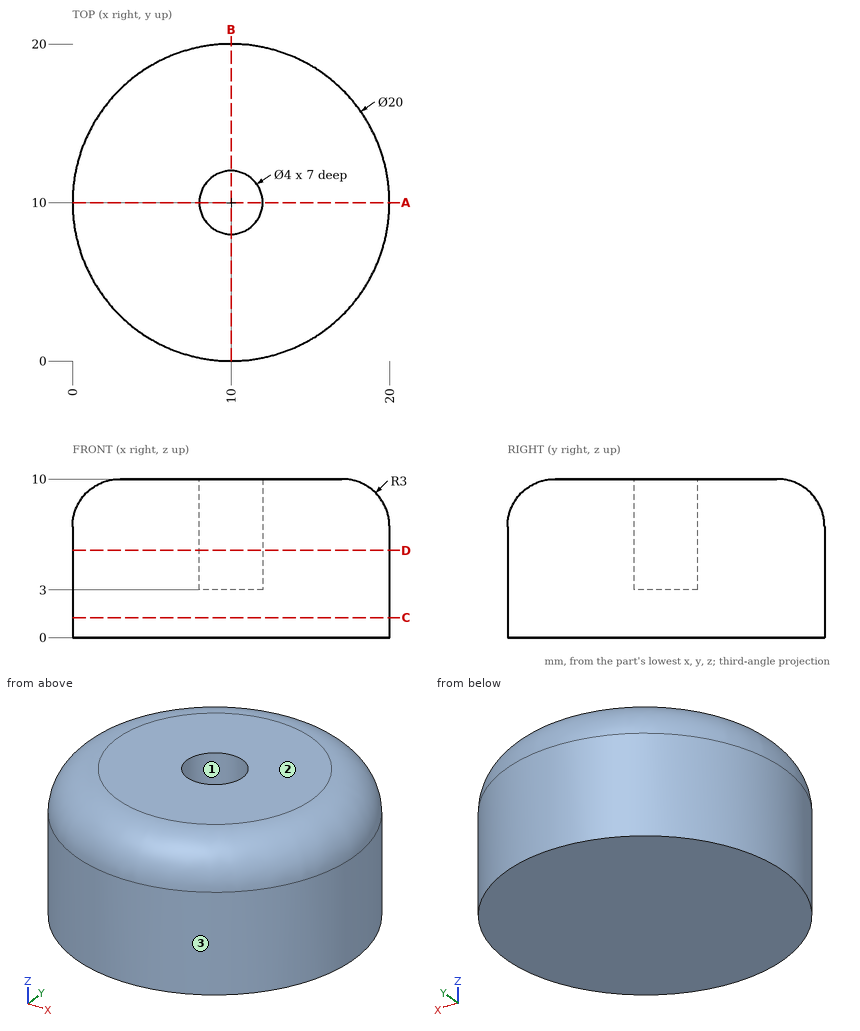
The figure shows three views and two pictorial views of one solid part (mm, origin at its lowest corner). Answer the questions. Round coordinates to 2 decimals unless told otherwise and drop trailing zeros. Write each loop counter-clockwise with the first axis right and the second up, starting at its lowest first coordinate (ties: lowest second). Pieces come first, ordered by that corner, then holes. Notation, with made-up numbers: M 49.5,34 L 60.5,34 A26 cw 60.5,51 Z; hole C -32.75,29.25 d3. An arc over 180 degrees is marked long. Use a Markdown table: item, result.
1) Consider line 1 (Y direction, x = 10, z = 4.5); line 2 (Y direction, x = 10, z = 8.5); line 3 (X direction, y = 9.75, z = 8.25). Determine where each line is inside the solid, lowest interval first. Write a range as [from, to].
Taken from the geometry:
| item | result |
|---|---|
| line 1 | y = [0, 8], [12, 20] |
| line 2 | y = [0.4, 8], [12, 19.6] |
| line 3 | x = [0.28, 8.02], [11.98, 19.72] |
2) The part is cut by section C-C on z = 1.25. Give the vertices of the cut face in (x, y), plus the area to 3 significant figures.
Taken from the geometry:
| item | result |
|---|---|
| outline | C 10,10 d20 |
| area | 314 mm2 |
3) Flat-ended cylindrical pins translate along their axes: pin 1 (10 mm diameter, centred on x = 14.5, y = 4.5, fed in from -Z); pin 2 (1 mm diameter, centred on y = 8, z = 1.5, fed in from -X); pin 3 (5 mm diameter, centred on x = 4, z = 2.5, fed in from +Y); pin 4 (6 mm diameter, centred on x = 5, z = 6.5, fed in from +Y). Find the tip coordinate at first contact, or state that the pin passes through.
Taken from the geometry:
| item | result |
|---|---|
| pin 1 | stops at z = 0 |
| pin 2 | stops at x = 0.11 |
| pin 3 | stops at y = 19.37 |
| pin 4 | stops at y = 19.8 |
4) Determine the mould class of the marked faces 1, 2 and 3 for opening direction X: pulls with the +X half, pulls with the -X half, needs draft (parallel to the pull), parting line crosses it, or undercut.
Taken from the geometry:
| item | result |
|---|---|
| face 1 | undercut |
| face 2 | needs draft |
| face 3 | parting line crosses it |
5) The part is cut by section A-A on y = 10. Give the vertices of the cut face in (x, z), plus the area to 3 significant figures.
Taken from the geometry:
| item | result |
|---|---|
| outline | M 0,0 L 20,0 L 20,7 A3 ccw 17,10 L 12,10 L 12,3 L 8,3 L 8,10 L 3,10 A3 ccw 0,7 Z |
| area | 168 mm2 |
6) The part is cut by section D-D on z = 5.5. Give the vertices of the cut face in (x, y).
Taken from the geometry:
| item | result |
|---|---|
| outline | C 10,10 d20; hole C 10,10 d4 |
